from build123d import *

# Parameters (mm, degrees)
SKETCH1_R           = 1.25
BOSS_EXTRUDE1_DEPTH = 20


with BuildPart() as part:
    # Sketch1 → Boss-Extrude1 (new body)
    with BuildSketch(Plane.XY):
        with BuildLine():
            Line((95.67108193, -66.01040764), (105.67108193, -56.01040764))
            ThreePointArc((105.67108193, -56.01040764), (107.513650317, -53.252809175), (108.16067429, -50))
            Line((108.16067429, -50), (108.16067429, -25))
            ThreePointArc((108.16067429, -25), (105.67108193, -18.98959236), (99.66067429, -16.5))
            Line((99.66067429, -16.5), (79.66067429, -16.5))
            ThreePointArc((79.66067429, -16.5), (73.65026665, -18.98959236), (71.16067429, -25))
            Line((71.16067429, -25), (71.16067429, -60))
            ThreePointArc((71.16067429, -60), (73.65026665, -66.01040764), (79.66067429, -68.5))
            Line((79.66067429, -68.5), (89.66067429, -68.5))
            ThreePointArc((89.66067429, -68.5), (92.913483465, -67.852976026), (95.67108193, -66.01040764))
        make_face()
        with Locations((73.41067429, -42.5)):
            Circle(SKETCH1_R, mode=Mode.SUBTRACT)
        with BuildLine():
            Line((104.963975149, -55.303300859), (101.554965407, -58.712310601))
            Line((101.554965407, -58.712310601), (100.67108193, -57.828427125))
            ThreePointArc((100.67108193, -57.828427125), (97.489101415, -57.828427125), (97.489101415, -61.01040764))
            Line((97.489101415, -61.01040764), (98.372984892, -61.894291117))
            Line((98.372984892, -61.894291117), (94.963975149, -65.303300859))
            ThreePointArc((94.963975149, -65.303300859), (92.530800033, -66.929096494), (89.66067429, -67.5))
            Line((89.66067429, -67.5), (79.66067429, -67.5))
            ThreePointArc((79.66067429, -67.5), (74.357373431, -65.303300859), (72.16067429, -60))
            Line((72.16067429, -60), (72.16067429, -44.75))
            Line((72.16067429, -44.75), (73.41067429, -44.75))
            ThreePointArc((73.41067429, -44.75), (75.66067429, -42.5), (73.41067429, -40.25))
            Line((73.41067429, -40.25), (72.16067429, -40.25))
            Line((72.16067429, -40.25), (72.16067429, -25))
            ThreePointArc((72.16067429, -25), (74.357373431, -19.696699141), (79.66067429, -17.5))
            Line((79.66067429, -17.5), (87.41067429, -17.5))
            Line((87.41067429, -17.5), (87.41067429, -18.75))
            ThreePointArc((87.41067429, -18.75), (89.66067429, -21), (91.91067429, -18.75))
            Line((91.91067429, -18.75), (91.91067429, -17.5))
            Line((91.91067429, -17.5), (99.66067429, -17.5))
            ThreePointArc((99.66067429, -17.5), (104.963975149, -19.696699141), (107.16067429, -25))
            Line((107.16067429, -25), (107.16067429, -40.25))
            Line((107.16067429, -40.25), (105.91067429, -40.25))
            ThreePointArc((105.91067429, -40.25), (103.66067429, -42.5), (105.91067429, -44.75))
            Line((105.91067429, -44.75), (107.16067429, -44.75))
            Line((107.16067429, -44.75), (107.16067429, -50))
            ThreePointArc((107.16067429, -50), (106.589770784, -52.870125743), (104.963975149, -55.303300859))
        make_face(mode=Mode.SUBTRACT)
        with Locations((89.66067429, -18.75)):
            Circle(SKETCH1_R, mode=Mode.SUBTRACT)
        with Locations((105.91067429, -42.5)):
            Circle(SKETCH1_R, mode=Mode.SUBTRACT)
        with Locations((99.080091673, -59.419417382)):
            Circle(SKETCH1_R, mode=Mode.SUBTRACT)
    extrude(amount=BOSS_EXTRUDE1_DEPTH)


solid = part.part
Input: part model. Units: mm. Frame: model coordinates. A direction names the side the tool comes from. Coordinates: 2 decimals unless noted, no trailing zeros. Order: outer loops, then holes, each group sorted by start corner. A loop starts at its lowest first (then second) coordinate and runs counter-clockwise, first axis right, second up. Notation, with made-up numbers: M 29.5,-1 L 47.5,-1 A16 ccw 47.5,5 Z; hole C 65.5,17 d8. An arc over 180 degrees is marked long. Answer in a Markdown table with one row per item.
(1) Section query A-A, the plane y = -47. Output: boundary loops of the cut face in (x, z), plus the area to 3 significant figures.
Numbers:
| item | result |
|---|---|
| outline | M 71.16,0 L 72.16,0 L 72.16,20 L 71.16,20 Z; M 107.16,0 L 108.16,0 L 108.16,20 L 107.16,20 Z |
| area | 40.0 mm^2 |
(2) Section query C-C, the plane z = 3. Give the number of separate pieces and of enclosed holes in the cut face, plus the area to 3 significant figures.
Numbers:
| item | result |
|---|---|
| separate pieces | 1 |
| enclosed holes | 5 |
| area | 189 mm^2 |
(3) Access query for faces 1 (the cylindrical face through (73.58, -65.94, 9.86)), 2 (the flat face through (107.161, -47, 10)). Directions: +Z, -Z, +X, -X, +Y, -Y. A direction counts if a zero-diameter tool reaches every point of the face in a straight line with its end or side. Return the directions, or none.
Numbers:
| item | result |
|---|---|
| face 1 | +Z, -Z, -X, -Y |
| face 2 | +Z, -Z |
(4) Contact query for flat-ended pins moving along their axis: pin 1 Ø4 at (x, z) = (92, 7) entering from -Y; pin 2 Ø0.6 at (x, z) = (106.5, 12.5) entering from -Y; pin 3 Ø2 at (x, y) = (99.08, -59.42) entering from +Z; pin 4 Ø8.5 at (x, z) = (97.5, 9) entering from -Y (3 decimals). Output: stop coordinate, or through.
Numbers:
| item | result |
|---|---|
| pin 1 | stops at y = -68.49 |
| pin 2 | stops at y = -55.43 |
| pin 3 | passes through |
| pin 4 | stops at y = -67.705 |
(5) Material intervals for line 1 (Y direction, x = 83, z = 3); line 2 (X direction, y = -37, z = 9.5); line 3 (X direction, y = -18.5, z = 11.25), sorted ascending. Write a range as [from, to].
Numbers:
| item | result |
|---|---|
| line 1 | y = [-68.5, -67.5], [-17.5, -16.5] |
| line 2 | x = [71.16, 72.16], [107.16, 108.16] |
| line 3 | x = [74.18, 75.92], [87.41, 88.44], [90.89, 91.91], [103.4, 105.14] |
(6) Draft query along Y for faces 3 (the flat face through (90, -16.5, 10)), 4 (the flat face through (71.161, -42, 10)), 5 (the cylindrical face through (97.524, -57.794, 9.86)), 6 (the cylindrical face through (89.6, -21, 9.9)). Return one class per face: pulls with the +Y half, pulls with the -Y half, needs draft (parallel to the pull), parting line crosses it, or undercut.
Numbers:
| item | result |
|---|---|
| face 3 | pulls with the +Y half |
| face 4 | needs draft |
| face 5 | undercut |
| face 6 | undercut |
(7) Section query B-B, the plane x = 85. Output: boundary loops of the cut face in (y, z).
Numbers:
| item | result |
|---|---|
| outline | M -68.5,0 L -67.5,0 L -67.5,20 L -68.5,20 Z; M -17.5,0 L -16.5,0 L -16.5,20 L -17.5,20 Z |
